Here's how the part is built. I have some questions about the finished solid (model axes, mm). Face numbers are marked on the shaded views. A direction names the side the tool comes from. Coordinates: 2 decimals unless noted, no trailing zeros. Order: outer loops, then holes, each group sorted by start corner. A loop starts at its lowest first (then second) coordinate and runs counter-clockwise, first axis right, second up. Notation, with made-up numbers: M 54.5,76 L 58.5,76 A26 cw 58.5,114 Z; hole C 87,-37.5 d3. An arc over 180 degrees is marked long. Answer as CSV lines item,"result". Start each with the question number.
Autodesk Fusion 360 part; units mm, degrees
sketch "Sketch1" plane through (0, 0, 0) normal (0, 0, 1) x (1, 0, 0)
  circle A0 centre (0, 0) radius 25.5
  line L0 (29.5, -30.5) -> (-29.5, -30.5)
  line L1 (-30.5, -29.5) -> (-30.5, 29.5)
  line L2 (-29.5, 30.5) -> (29.5, 30.5)
  line L3 (30.5, 29.5) -> (30.5, -29.5)
  line L4 (30.5, -30.5) -> (-30.5, 30.5) construction
  line L5 (-30.5, -30.5) -> (30.5, 30.5) construction
  arc A1 (-29.5, 30.5) -> (-30.5, 29.5) centre (-29.5, 29.5) ccw
  arc A2 (30.5, 29.5) -> (29.5, 30.5) centre (29.5, 29.5) ccw
  arc A3 (29.5, -30.5) -> (30.5, -29.5) centre (29.5, -29.5) ccw
  arc A4 (-30.5, -29.5) -> (-29.5, -30.5) centre (-29.5, -29.5) ccw
  line L6 (48, -50) -> (-48, -50)
  line L7 (-50, -48) -> (-50, 48)
  line L8 (-48, 50) -> (48, 50)
  line L9 (50, 48) -> (50, -48)
  line L10 (50, -50) -> (-50, 50) construction
  line L11 (-50, -50) -> (50, 50) construction
  arc A5 (-48, 50) -> (-50, 48) centre (-48, 48) ccw
  arc A6 (50, 48) -> (48, 50) centre (48, 48) ccw
  arc A7 (48, -50) -> (50, -48) centre (48, -48) ccw
  arc A8 (-50, -48) -> (-48, -50) centre (-48, -48) ccw
  line L12 (0, -30.5) -> (22, -30.5)
  line L13 (22, -30.5) -> (22, 30.5)
  line L14 (22, 30.5) -> (0, 30.5)
  line L15 (0, 30.5) -> (0, -30.5)
  line L16 (-22, -30.5) -> (-22, 30.5)
  line L17 (-30.5, 0) -> (-30.5, 22)
  line L18 (-30.5, 22) -> (30.5, 22)
  line L19 (-30.5, 22) -> (30.5, 22)
  line L20 (30.5, 22) -> (30.5, -22)
  line L21 (30.5, -22) -> (-30.5, -22)
  line L22 (-30.5, -22) -> (-30.5, 22)
  dimension "d1" = 51
  dimension "d2" = 61
  dimension "d3" = 61
  dimension "d4" = 1
  dimension "d5" = 1
  dimension "d6" = 1
  dimension "d7" = 1
  dimension "d8" = 100
  dimension "d9" = 100
  dimension "d14" = 2
  dimension "d15" = 2
  dimension "d16" = 2
  dimension "d17" = 2
  dimension "d18" = 22
  dimension "d19" = 22
  dimension "d20" = 61
  dimension "d21" = 44
extrude "Extrude1" add sketch "Sketch1" along normal blind 130 contours A0 L3 L13 L18 L19 L20 L21 | A0 L13 L18 L19 | A0 L13 L21 | A0 L2 L13 L14 L15 L18 L19 | L2 L3 A2 L13 L18 L19 | A0 L0 L12 L13 L15 L21 | L0 L3 A3 L13 L21 | A0 L2 L15 L16 L18 L19 | A0 L0 L15 L16 L21 | A0 L16 L18 L19 | A0 L16 L21 | A0 L1 L16 L17 L18 L19 L21 L22 | L1 L2 A1 L16 L18 L19 | L0 L1 A4 L16 L21
extrude "Extrude2" add sketch "Sketch1" against normal blind 5 contours A0 L13 | A0 L3 L13 L18 L19 L20 L21 | A0 L13 L15 L18 L19 L21 | A0 L13 L18 L19 | A0 L13 L21 | A0 L15 L18 L19 | A0 L2 L13 L14 L15 L18 L19 | L2 L3 A2 L13 L18 L19 | A0 L0 L12 L13 L15 L21 | A0 L15 L21 | L0 L3 A3 L13 L21 | A0 L15 L18 L19 | A0 L2 L15 L16 L18 L19 | A0 L15 L16 L18 L19 L21 | A0 L0 L15 L16 L21 | A0 L15 L21 | A0 L16 L18 L19 | A0 L16 L21 | A0 L16 | A0 L1 L16 L17 L18 L19 L21 L22 | L1 L2 A1 L16 L18 L19 | L0 L1 A4 L16 L21 | L6 L7 L8 L9 A5 A6 A7 A8
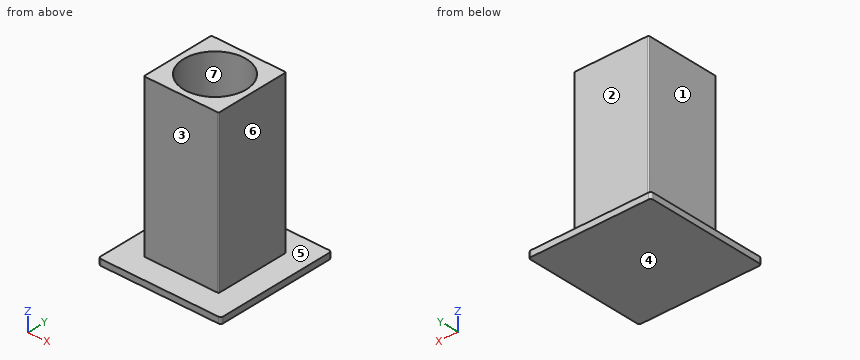
1) Suppose I cut it at A-A on z = 38.5. Please give me the cut outline in (x, y).
2) Which directions (+Z, -Z, +X, -X, +Y, -Y) give clear straight access to the entire face, cutting with the end or side of a thin tool? Please do the marked faces 1, 2, 3 and 4.
3) If we mould it in two halves opening along X, with no side actions, what happens to the marked faces 5, 6 and 7? For each: released by +X, released by -X, zero draft, split by the parting line, or undercut.
4) Suppose I cut it at D-D on y = -44. Please give me the cut outline in (x, z), plus the area to 3 significant figures.
5) I need wall thicknesses on line 1 (X direction, y = 0, z = 44); line 2 (Z direction, x = 44.5, y = -38). Which ranges of each line are inside material? Lowest first, please. Write a range as [from, to].
6) Suppose I cut it at B-B on x = 0. Please give me the cut outline in (y, z), plus the area to 3 significant figures.
7) Will these pins go through, and if not, where does the flat tip stop? pin 1 Ø6 at (y, z) = (-27.5, 21.5) entering from +X; pin 2 Ø1.5 at (x, z) = (-13, 31) entering from +Y; pin 3 Ø5 at (x, z) = (-18.5, 96.5) entering from -Y.
Output:
1,outline,"M -30.5,-29.5 A1 ccw -29.5,-30.5 L 29.5,-30.5 A1 ccw 30.5,-29.5 L 30.5,29.5 A1 ccw 29.5,30.5 L -29.5,30.5 A1 ccw -30.5,29.5 Z; hole C 0,0 d51"
2,face 1,"+Z, -X, +Y, -Y"
2,face 2,"+Z, +X, -X, +Y"
2,face 3,"+Z, +X, -X, -Y"
2,face 4,"-Z, +X, -X, +Y, -Y"
3,face 5,"zero draft"
3,face 6,"released by +X"
3,face 7,"undercut"
4,outline,"M -50,-5 L 50,-5 L 50,0 L -50,0 Z"
4,area,"500 mm²"
5,line 1,"[-30.5, -25.5], [25.5, 30.5]"
5,line 2,"[-5, 0]"
6,outline,"M -50,-5 L 50,-5 L 50,0 L 30.5,0 L 30.5,130 L 25.5,130 L 25.5,0 L -25.5,0 L -25.5,130 L -30.5,130 L -30.5,0 L -50,0 Z"
6,area,"1,800 mm²"
7,pin 1,"x = 30.5"
7,pin 2,"y = 30.5"
7,pin 3,"y = -30.5"
